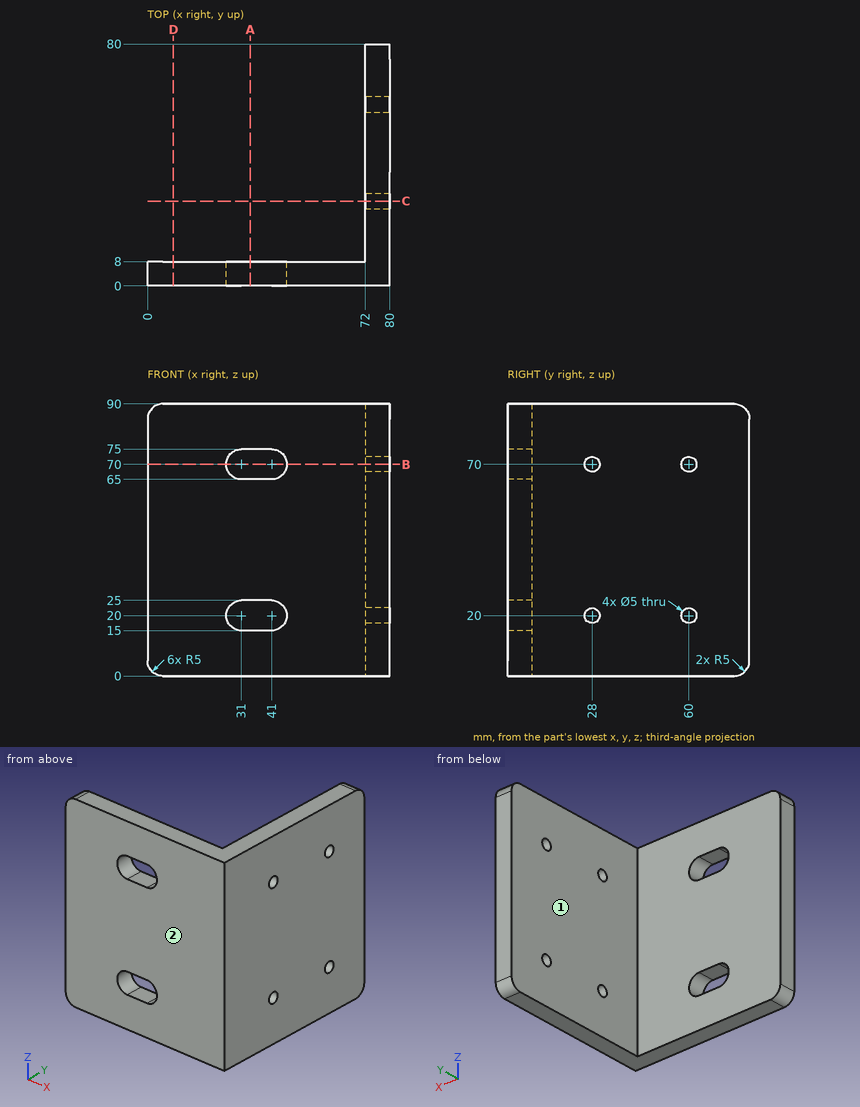
The drawing under review shows one solid part. Ordinate dimensions are in mm from its lowest x, y, z. A direction names the side the tool comes from. Round coordinates to 2 decimals unless told otherwise and drop trailing zeros. Order: outer loops, then holes, each group sorted by start corner. A loop starts at its lowest first (then second) coordinate and runs counter-clockwise, first axis right, second up. Notation, with made-up numbers: (39.5, 26) -> (89.5, 26) arc R25 ccw to (89.5, 41) -> close; hole circle Ø8 at (-39.5, -16). An arc over 180 degrees is marked (long way). Return JSON: item names as keys, results as strings.
1. Take a section at B-B (z = 70). Write out the cut boundary in (x, y), then the cut area to 3 significant figures.
Answer block:
{"outline": "(0, 0) -> (26, 0) -> (26, 8) -> (0, 8) -> close; (46, 0) -> (80, 0) -> (80, 25.5) -> (72, 25.5) -> (72, 8) -> (46, 8) -> close; (72, 30.5) -> (80, 30.5) -> (80, 57.5) -> (72, 57.5) -> close; (72, 62.5) -> (80, 62.5) -> (80, 80) -> (72, 80) -> close", "area": "976 mm²"}
2. For the marked faces 1 and 2, list the 3-axis set-ups (+Z, -Z, +X, -X, +Y, -Y) from which the entire face can be reached by the end or side of a thin tool; tool diameter is ignored.
Answer block:
{"face 1": "+Z, -Z, -X, +Y", "face 2": "+Z, -Z, +X, -X, -Y"}
3. Take a section at D-D (x = 8.5). Write out the cut boundary in (y, z).
Answer block:
{"outline": "(0, 0) -> (8, 0) -> (8, 90) -> (0, 90) -> close"}
4. Insertion check: P1, Ø4, axis at x = 30.5, z = 79, coming from the +Y side; P2, Ø6, axis at y = 28, z = 70, coming from the -X side. Each pin has a flat end and moves straight along its axis. Give the tip position at first contact, or say it passes through.
Answer block:
{"P1": "stops at y = 8", "P2": "stops at x = 72"}
5. For L1, parallel to Z at x = 78, y = 60; L2, parallel to Y at x = 76, z = 70; L3, parallel to Y at x = 25, z = 66, list the stretches that pass through material, from the lowest coordinate up. Write a range as [from, to].
Answer block:
{"L1": "z = [0, 17.5], [22.5, 67.5], [72.5, 90]", "L2": "y = [0, 25.5], [30.5, 57.5], [62.5, 80]", "L3": "y = [0, 8]"}
6. Take a section at A-A (x = 34). Write out the cut boundary in (y, z), then the cut area to 3 significant figures.
Answer block:
{"outline": "(0, 0) -> (8, 0) -> (8, 15) -> (0, 15) -> close; (0, 25) -> (8, 25) -> (8, 65) -> (0, 65) -> close; (0, 75) -> (8, 75) -> (8, 90) -> (0, 90) -> close", "area": "560 mm²"}
7. Take a section at C-C (y = 28). Write out the cut boundary in (x, z), then the cut area to 3 significant figures.
Answer block:
{"outline": "(72, 0) -> (80, 0) -> (80, 17.5) -> (72, 17.5) -> close; (72, 22.5) -> (80, 22.5) -> (80, 67.5) -> (72, 67.5) -> close; (72, 72.5) -> (80, 72.5) -> (80, 90) -> (72, 90) -> close", "area": "640 mm²"}
